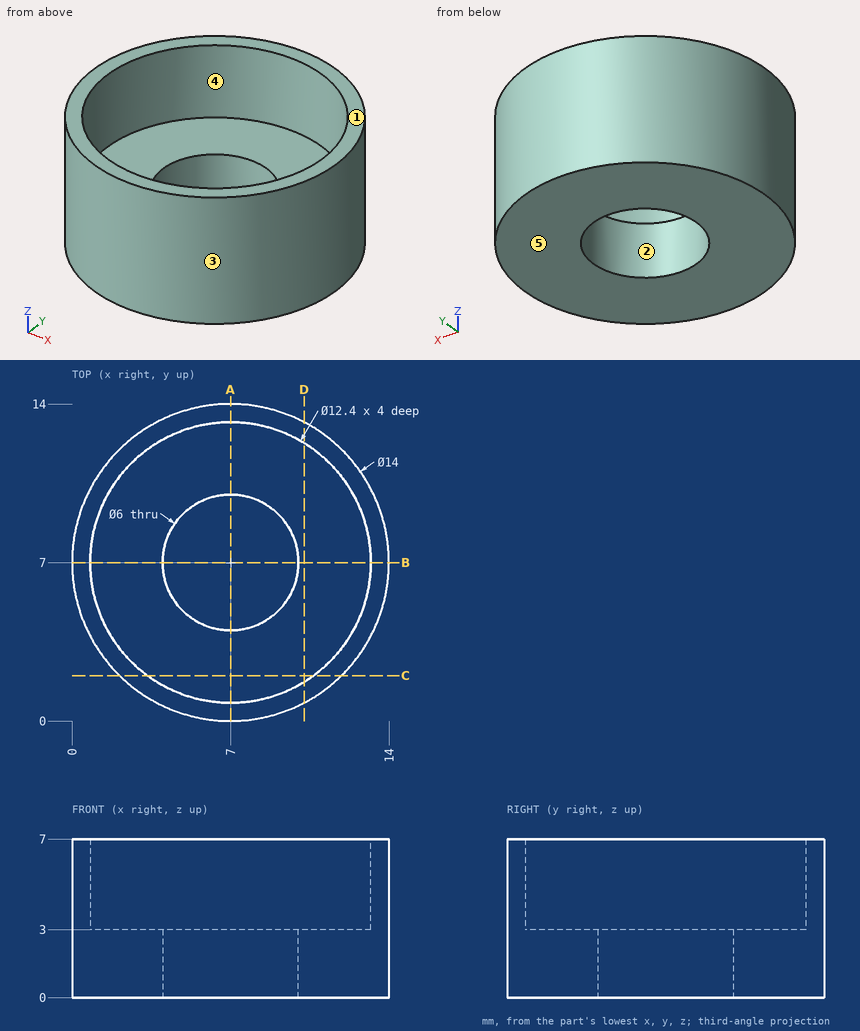
The figure shows three views and two pictorial views of one solid part (mm, origin at its lowest corner). Answer the questions. A direction names the side the tool comes from. Round coordinates to 2 decimals unless told otherwise and drop trailing zeros. Loops run counter-clockwise (first coordinate to the right, second up) from the corner with the lowest first, then second, coordinate; pieces in that order, holes last. Notation, with made-up numbers: (53, 80.5) -> (66, 80.5) arc R30 ccw to (66, 118.5) -> close; hole circle Ø10 at (-30.75, 43). An arc over 180 degrees is marked (long way). Use one line per item in the form item = value.
(1) Flat-ended cylindrical pins translate along their axes: P1, Ø1.5, axis at x = 9.5, z = 4.5, coming from the +Y side; P2, Ø1.5, axis at y = 9, z = 1.5, coming from the -X side. Find the tip coordinate at first contact, or state that the pin passes through.
Answer list:
P1 = 13.78
P2 = 0.11
(2) Find section A-A on x = 7. Give the vertices of the cut face in (y, z).
Answer list:
outline = (0, 0) -> (4, 0) -> (4, 3) -> (0.8, 3) -> (0.8, 7) -> (0, 7) -> close; (10, 0) -> (14, 0) -> (14, 7) -> (13.2, 7) -> (13.2, 3) -> (10, 3) -> close
(3) A tool of negligible diameter and unlimited length cuts with its end or side. For the marked faces 4 and 5, from which of +Z, -Z, +X, -X, +Y, -Y can it reach the whole face along a straight path? Write none if from no direction.
Answer list:
face_4 = +Z
face_5 = -Z, +X, -X, +Y, -Y
(4) For a pull along Y with two mould halves and no side action, classify the marked faces 1, 2 and 3 as released by +Y, released by -Y, zero draft, split by the parting line, or undercut.
Answer list:
face_1 = zero draft
face_2 = undercut
face_3 = split by the parting line
(5) Find section D-D on x = 10.25. Give the vertices of the cut face in (y, z), then the cut area to 3 significant figures.
Answer list:
outline = (0.8, 0) -> (13.2, 0) -> (13.2, 7) -> (12.28, 7) -> (12.28, 3) -> (1.72, 3) -> (1.72, 7) -> (0.8, 7) -> close
area = 44.6 mm2
(6) Straight lines are drawn through the part: line 1 (Y direction, x = 7, z = 2.15); line 2 (Z direction, x = 9.25, y = 2.5); line 3 (Y direction, x = 2.5, z = 5). For each, find the intervals that lie inside material, in ascending order.
Answer list:
line_1 = 0 to 4, 10 to 14
line_2 = 0 to 3
line_3 = 1.64 to 2.74, 11.26 to 12.36
(7) Find section C-C on y = 2. Give the vertices of the cut face in (x, z).
Answer list:
outline = (2.1, 0) -> (11.9, 0) -> (11.9, 7) -> (10.67, 7) -> (10.67, 3) -> (3.33, 3) -> (3.33, 7) -> (2.1, 7) -> close
